Verification items for the finished model (mm, model axes). Face numbers are marked on the shaded views. Round coordinates to 2 decimals unless told otherwise and drop trailing zeros. Order: outer loops, then holes, each group sorted by start corner. A loop starts at its lowest first (then second) coordinate and runs counter-clockwise, first axis right, second up. Notation, with made-up numbers: (-36, -28) -> (22, -28) arc R20 cw to (22, -23) -> close; hole circle Ø8 at (34.5, -8). An arc over 180 degrees is marked (long way). Return JSON: item names as keys, results as strings. Group by question number.
1) Section check A-A on y = -1. Enter the section's corners in (x, z).
2) Draft check along X on the marked faces 1, 2 and 3. Enter one of: pulls with the +X half, pulls with the -X half, needs draft (parallel to the pull), parting line crosses it, or undercut.
3) Section check C-C on z = 14.5. Enter the section's corners in (x, y), plus the area to 3 significant figures.
4) Scan lines: L1, parallel to X at y = 0, z = 2.5 (3 decimals); L2, parallel to X at y = 0, z = 15. Record each from-to range of solid material in increasing order.
5) Depth check by flat-ended pin: pin 1 (2 mm diameter, centred on y = -1.5, z = 13, fed in from +X); pin 2 (4 mm diameter, centred on x = 4.5, z = 11.5, fed in from -Y); pin 3 (1 mm diameter, centred on y = -3.5, z = 13, fed in from -X). Enter the tip coordinate at first touch or a pass-through.
6) Section check B-B on z = 1. Enter the section's corners in (x, y) (3 decimals), plus the area to 3 significant figures.
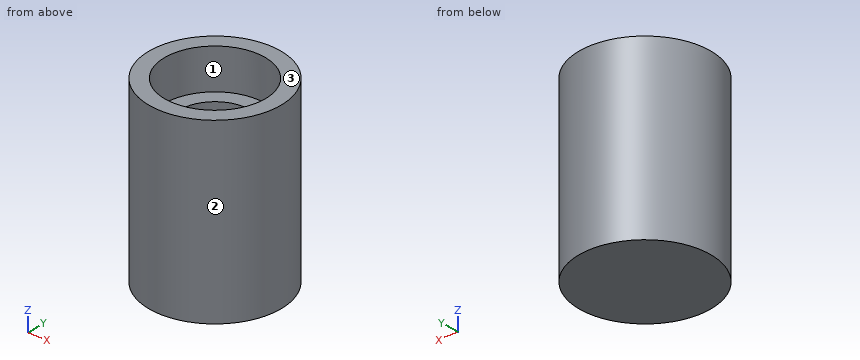
Autodesk Fusion 360 part; units mm, degrees
sketch "Sketch1" plane through (0, 0, 0) normal (0, 0, 1) x (1, 0, 0)
  circle A0 centre (0, 0) radius 5.9
  dimension "d1" = 11.8
extrude "Extrude1" add sketch "Sketch1" along normal blind 15
sketch "Sketch2" plane through (0, 0, 0) normal (0, 0, 1) x (1, 0, 0)
sketch "Sketch3" plane through (0, 0, 15) normal (0, 0, 1) x (-1, 0, 0)
  circle A0 centre (0, 0) radius 5.9
  circle A1 centre (0, 0) radius 4.5
  dimension "d4" = 9
extrude "Extrude2" add sketch "Sketch3" along normal blind 1
extrude "Extrude3" cut 1 faces at (-0.5857, 1.1465, 15) along direction (0, 0, -1) blind 2.6
sketch "Sketch4" plane through (0, 0, 12.4) normal (0, 0, 1) x (-1, 0, 0)
  circle A0 centre (0, 0) radius 4.5
  circle A1 centre (0, 0) radius 3.125
  dimension "d9" = 6.25
extrude "Extrude4" cut sketch "Sketch4" against normal blind 12 contours A1
Check result:
{
 "1": {"outline": "(-5.81, 0) -> (5.81, 0) -> (5.81, 16) -> (4.39, 16) -> (4.39, 12.4) -> (2.96, 12.4) -> (2.96, 0.4) -> (-2.96, 0.4) -> (-2.96, 12.4) -> (-4.39, 12.4) -> (-4.39, 16) -> (-5.81, 16) -> close"},
 "2": {"face 1": "undercut", "face 2": "parting line crosses it", "face 3": "needs draft"},
 "3": {"outline": "circle Ø11.8 at (0, 0); hole circle Ø9 at (0, 0)", "area": "45.7 mm^2"},
 "4": {"L1": "-5.9 to -3.125, 3.125 to 5.9", "L2": "-5.9 to -4.5, 4.5 to 5.9"},
 "5": {"pin 1": "x = 5.88", "pin 2": "y = -5.34", "pin 3": "x = -5.08"},
 "6": {"outline": "circle Ø11.8 at (0, 0); hole circle Ø6.25 at (0, 0)", "area": "78.7 mm^2"}
}
